Part model, mm, in its own coordinate system. Face numbers are marked on the shaded views. A direction names the side the tool comes from. Round coordinates to 2 decimals unless told otherwise and drop trailing zeros. Loops run counter-clockwise (first coordinate to the right, second up) from the corner with the lowest first, then second, coordinate; pieces in that order, holes last.
(1) Flat gauge pins, fed straight in: pin 1 (3 mm diameter, centred on x = -9.5, y = 3, fed in from -Z); pin 2 (4.5 mm diameter, centred on x = 0, z = 46, fed in from +Y); pin 3 (3 mm diameter, centred on x = 27.5, y = 38, fed in from -Z). Where does each tip first touch, or does it go through?
(2) Cut at A-A on y = 27. List the corners of the cut face in (x, z).
(3) Cut at C-C on z = 0. List the corners of the cut face in (x, y).
(4) Probe probe 1 along Z at (x, y) = (0, 37); probe 2 along Z at (x, y) = (0, -8.15); probe 3 along Y at (x, z) = (3.5, -23.5). List the from-to ranges inside material, lowest first.
(5) Tool access for the marked faces 1, 2 and 3: list every direction of +Z, -Z, +X, -X, +Y, -Y with a clear straight run to the whole face (end or side of a thin tool).
(6) Mould opens along Z. For the marked faces 4, 5, 6 and 7 say: +Z half, -Z half, draft (parallel to the pull), parting line (faces both ways), or undercut.
from build123d import *

# Parameters (mm, degrees)
F2_R     = 2
F5_W     = 7
F5_H     = 50
F6_DEPTH = 20
F8_R     = 5
F7_W     = 38
F7_H     = 11
F9_DEPTH = 25


# Not quite as in the source:
# - a fillet or chamfer that OpenCascade refuses, or shapes differently, is made with other operations: its cross-section is extruded or revolved along the edge and cut away or added
# - two fillets or chamfers of one size are made in one step


with BuildPart() as f1:
    # F0 (on Top) → F1 (revolve)
    with BuildSketch(Plane.XY):
        Polygon((0, -7), (0, 0), (-30, 0), (-30, 77), (-37, 77), (-37, -7), (-34, -7), (-34, -9), (-27, -9), (-27, -7), align=None)
    revolve(axis=Axis((0, 38.5, 0), (0, 1, 0)))

    # F2
    f2_edges = [f1.edges().sort_by_distance(p)[0] for p in [
        (37, 77, 0),
        (30, 77, 0),
    ]]
    fillet(f2_edges, radius=F2_R)

    # F3: fillet of radius 5 on 1 edges, made by hand

    # F3_s1 → F3_t2 (revolve, cut)
    with BuildSketch(Plane.XY):
        with BuildLine():
            ThreePointArc((-37, -2.417424305), (-36.1833001327, -5.1560370926), (-34, -7))
            Line((-34, -7), (-37, -7))
            Line((-37, -7), (-37, -2.417424305))
        make_face()
    revolve(axis=Axis((0, -7, 0), (0, 1, 0)), mode=Mode.SUBTRACT)

    # F5 (on offset) → F6 (join)
    with BuildSketch(Plane.XY.offset(35)):
        with Locations((-3.5, 40)):
            Rectangle(F5_W, F5_H)
        with Locations((3.5, 40)):
            Rectangle(F5_W, F5_H)
    extrude(amount=F6_DEPTH)

    # F8
    f8_edges = [f1.edges().sort_by_distance(p)[0] for p in [
        (0, 65, 55),
        (0, 15, 55),
        (7, 15, 45.665902),
        (-7, 15, 45.665902),
        (-7, 40, 55),
        (-7, 65, 45.665902),
        (7, 65, 45.665902),
        (7, 40, 55),
    ]]
    fillet(f8_edges, radius=F8_R)

    # F7 (on face) → F9 (cut)
    with BuildSketch(Plane.YZ.offset(7)):
        with Locations((40, 43.5)):
            Rectangle(F7_W, F7_H)
    extrude(amount=-F9_DEPTH, mode=Mode.SUBTRACT)


solid = f1.part
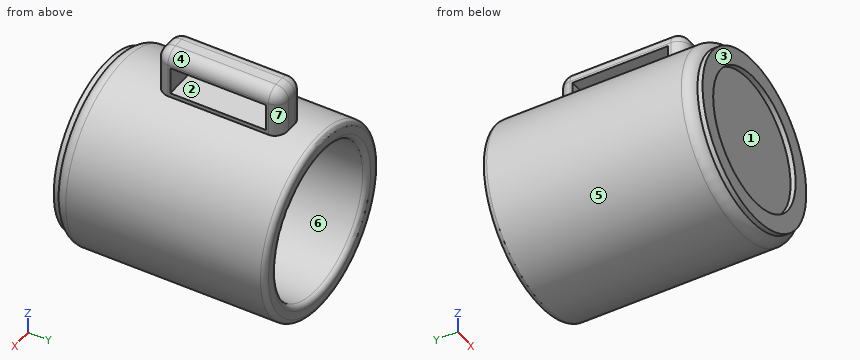
Final values:
1. pin 1: stops at z = -36.12
1. pin 2: stops at y = 65
1. pin 3: stops at z = -26.32
2. outline: (-7, 36.33) arc R37 ccw (long way) to (7, 36.33) - (7, 38) - (-7, 38) - close; (-7, 49) - (7, 49) - (7, 50) arc R5 ccw to (2, 55) - (-2, 55) arc R5 ccw to (-7, 50) - close; hole circle Ø60 at (0, 0)
3. outline: (-37, -2.42) arc R5 ccw to (-34, -7) - (-34, -9) - (-27, -9) - (-27, -7) - (27, -7) - (27, -9) - (34, -9) - (34, -7) arc R5 ccw to (37, -2.42) - (37, 75) arc R2 ccw to (35, 77) - (32, 77) arc R2 ccw to (30, 75) - (30, 0) - (-30, 0) - (-30, 75) arc R2 ccw to (-32, 77) - (-35, 77) arc R2 ccw to (-37, 75) - close
4. probe 1: z = -37 to -30, 30 to 38, 49 to 55
4. probe 2: z = -34 to -27, 27 to 34
4. probe 3: y = -7 to 0
5. face 1: -Y
5. face 2: +X, -X
5. face 3: +Z, -Z, +X, -X, -Y
6. face 4: +Z half
6. face 5: parting line
6. face 6: undercut
6. face 7: draft
